```python
from build123d import *

# Parameters (mm, degrees)
SKETCH1_W           = 18
SKETCH1_H           = 18
SKETCH1_R           = 1.625
BOSS_EXTRUDE1_DEPTH = 4
SKETCH2_W           = 1
SKETCH2_H           = 6
CUT_EXTRUDE1_DEPTH  = 0.95
SKETCH3_R           = 1.625
BOSS_EXTRUDE2_DEPTH = 0.5
FILLET1_R           = 1


with BuildPart() as part:
    # Sketch1 → Boss-Extrude1 (new body)
    with BuildSketch(Plane.XY):
        with Locations((9, 9)):
            Rectangle(SKETCH1_W, SKETCH1_H)
        with Locations((4, 4)):
            Circle(SKETCH1_R, mode=Mode.SUBTRACT)
        with Locations((14, 4)):
            Circle(SKETCH1_R, mode=Mode.SUBTRACT)
        with Locations((14, 14)):
            Circle(SKETCH1_R, mode=Mode.SUBTRACT)
    extrude(amount=BOSS_EXTRUDE1_DEPTH)

    # Sketch2 → Cut-Extrude1 (cut)
    with BuildSketch(Plane(origin=(0, 0, 0), x_dir=(-1, 0, 0), z_dir=(0, 0, -1))):
        with Locations((-17.5, 9)):
            Rectangle(SKETCH2_W, SKETCH2_H)
        with Locations((-15.5, 9)):
            Rectangle(SKETCH2_W, SKETCH2_H)
        with Locations((-13.5, 9)):
            Rectangle(SKETCH2_W, SKETCH2_H)
        with Locations((-11.5, 9)):
            Rectangle(SKETCH2_W, SKETCH2_H)
        with Locations((-9.5, 9)):
            Rectangle(SKETCH2_W, SKETCH2_H)
        with Locations((-7.5, 9)):
            Rectangle(SKETCH2_W, SKETCH2_H)
        with Locations((-5.5, 9)):
            Rectangle(SKETCH2_W, SKETCH2_H)
        with Locations((-3.5, 9)):
            Rectangle(SKETCH2_W, SKETCH2_H)
        with Locations((-1.5, 9)):
            Rectangle(SKETCH2_W, SKETCH2_H)
    extrude(amount=-CUT_EXTRUDE1_DEPTH, mode=Mode.SUBTRACT)

    # Sketch3 → Boss-Extrude2 (add)
    with BuildSketch(Plane(origin=(0, 0, 0), x_dir=(-1, 0, 0), z_dir=(0, 0, -1))):
        Polygon((0, 0), (0, 6), (-1, 6), (-2, 6), (-3, 6), (-4, 6), (-5, 6), (-6, 6), (-7, 6), (-8, 6), (-9, 6), (-10, 6), (-11, 6), (-12, 6), (-13, 6), (-14, 6), (-15, 6), (-16, 6), (-17, 6), (-18, 6), (-18, 0), align=None)
        with Locations((-14, 4)):
            Circle(SKETCH3_R, mode=Mode.SUBTRACT)
        with Locations((-4, 4)):
            Circle(SKETCH3_R, mode=Mode.SUBTRACT)
        Polygon((0, 18), (-18, 18), (-18, 12), (-17, 12), (-16, 12), (-15, 12), (-14, 12), (-13, 12), (-12, 12), (-11, 12), (-10, 12), (-9, 12), (-8, 12), (-7, 12), (-6, 12), (-5, 12), (-4, 12), (-3, 12), (-2, 12), (-1, 12), (0, 12), align=None)
        with Locations((-14, 14)):
            Circle(SKETCH3_R, mode=Mode.SUBTRACT)
    extrude(amount=BOSS_EXTRUDE2_DEPTH)

    # Fillet1
    fillet1_edges = [part.edges().sort_by_distance(p)[0] for p in [
        (0, 18, 1.75),
        (18, 18, 1.75),
        (18, 0, 1.75),
        (0, 0, 1.75),
    ]]
    fillet(fillet1_edges, radius=FILLET1_R)


with BuildPart() as body_2:
    # Mirror1: mirrored copy
    add(part.part.mirror(Plane(origin=(18, 0, 4), x_dir=(0, 0, 1), z_dir=(-1, 0, 0))))


solid = body_2.part
```
Verification items for the finished model (mm, model axes). A direction names the side the tool comes from. Give positions to 0.01 mm unless a question says otherwise; leave off trailing zeros. Loops run counter-clockwise (first coordinate to the right, second up) from the corner with the lowest first, then second, coordinate; pieces in that order, holes last. Notation, with made-up numbers: M -18.5,50 L 2.5,50 A12 cw 2.5,55 Z; hole C -20,-20 d11. An arc over 180 degrees is marked long. Return JSON: item names as keys, results as strings.
1) Tool access check on faces 1 (the flat face through (35.5, 9, 0)), 2 (the flat face through (27, 9, 0.5)), 3 (the flat face through (27, 3, -0.5)). Record the directions out of +Z, -Z, +X, -X, +Y, -Y that give a thin tool (end or side, any length) a straight path to the whole face; none if there is none.
Findings:
{"face 1": "-Z, +X, -X", "face 2": "-Z", "face 3": "-Z, +X, -X, +Y, -Y"}
2) Section check C-C, the plane z = 3.75. Enter the section's corners in (x, y) (3 decimals), and give its area (3 significant figures).
Findings:
{"outline": "M 18,1 A1 ccw 19,0 L 35,0 A1 ccw 36,1 L 36,17 A1 ccw 35,18 L 19,18 A1 ccw 18,17 Z; hole C 22,4 d3.25; hole C 22,14 d3.25; hole C 32,4 d3.25", "area": "298 mm2"}
3) Material ranges on L1, parallel to X at y = 4, z = 2.75 (3 decimals); L2, parallel to Y at x = 32, z = -0.2 (3 decimals); L3, parallel to X at y = 14, z = 2.9 (3 decimals), recorded low to high. Write a range as [from, to].
Findings:
{"L1": "x = [18, 20.375], [23.625, 30.375], [33.625, 36]", "L2": "y = [0, 2.375], [5.625, 6], [12, 18]", "L3": "x = [18, 20.375], [23.625, 36]"}
4) Section check D-D, the plane x = 29.25. Enter the section's corners in (y, z), and give its area (3 significant figures).
Findings:
{"outline": "M 0,-0.5 L 6,-0.5 L 6,0 L 12,0 L 12,-0.5 L 18,-0.5 L 18,4 L 0,4 Z", "area": "78.0 mm2"}
5) Section check A-A, the plane y = 14. Enter the section's corners in (x, z) (3 decimals), and give its area (3 significant figures).
Findings:
{"outline": "M 18,-0.5 L 20.375,-0.5 L 20.375,4 L 18,4 Z; M 23.625,-0.5 L 36,-0.5 L 36,4 L 23.625,4 Z", "area": "66.4 mm2"}
6) Mould release check, pull along X, two halves, no side actions. Record for faces 4 (the flat face through (28.5, 9, 0.95)), 5 (the cylindrical face through (35.715, 17.699, 1.719)), 6 (the flat face through (18.5, 9, 0.95)): released by +X, released by -X, zero draft, split by the parting line, or undercut.
Findings:
{"face 4": "undercut", "face 5": "released by +X", "face 6": "zero draft"}
7) Gauge pin test, flat ends, axial feed: P1, Ø4, axis at x = 22.5, y = 12.5, coming from the -Z side; P2, Ø1.1, axis at x = 33.5, y = 9.5, coming from the -Z side; P3, Ø0.5, axis at y = 9.5, z = 0.5, coming from the -X side; P4, Ø0.8, axis at x = 24.5, y = 8, coming from the -Z side. Record the tip position at first contact, or that the pin passes through.
Findings:
{"P1": "stops at z = -0.5", "P2": "stops at z = 0", "P3": "stops at x = 19", "P4": "stops at z = 0.95"}
8) Section check B-B, the plane y = 4. Enter the section's corners in (x, z) (3 decimals).
Findings:
{"outline": "M 18,-0.5 L 20.375,-0.5 L 20.375,4 L 18,4 Z; M 23.625,-0.5 L 30.375,-0.5 L 30.375,4 L 23.625,4 Z; M 33.625,-0.5 L 36,-0.5 L 36,4 L 33.625,4 Z"}
